Verification items for this drawing (mm, ordinates from the low corner). A direction names the side the tool comes from. Coordinates: 2 decimals unless noted, no trailing zeros. Order: outer loops, then holes, each group sorted by start corner. A loop starts at its lowest first (then second) coordinate and runs counter-clockwise, first axis right, second up. Notation, with made-up numbers: M 6,-8 L 48,-8 A14 ccw 48,16 Z; hole C 26,1.25 d7. An arc over 180 degrees is marked long. One line per item, written item: value. Start each with the question number.
1) Go/stop test with flat-tipped pins: P1, Ø6, axis at y = 17.5, z = 12.5, coming from the +X side; P2, Ø5, axis at x = 3, y = 5, coming from the +Z side; P3, Ø3, axis at y = 18.5, z = 7, coming from the -X side. Record where each tip stops, or that it passes through.
2) Sectioned sample at C-C, the plane y = 15. Enter the section's corners in (x, z).
3) Access from +Z, -Z, +X, -X, +Y, -Y to the whole of each face (thin tool, end or side, straight path). Record for the marked faces 1, 2, 3, 4 and 5.
4) Sectioned sample at A-A, the plane y = 31. Enter the section's corners in (x, z), then the cut area to 3 significant figures.
5) Draft check along X on the marked faces 6, 7 and 8. Enter one of: pulls with the +X half, pulls with the -X half, needs draft (parallel to the pull), parting line crosses it, or undercut.
6) Sectioned sample at B-B, the plane x = 3. Enter the section's corners in (y, z), then the cut area to 3 significant figures.
7) Thickness scan on L1, parallel to Y at x = 34, z = 0.8; L2, parallel to X at y = 2, z = 19; L3, parallel to X at y = 2, z = 2. Record the ranges inside material, lowest first. Write a range as from..to.
8) Sectioned sample at D-D, the plane z = 6.25. Enter the section's corners in (x, y), then the cut area to 3 significant figures.
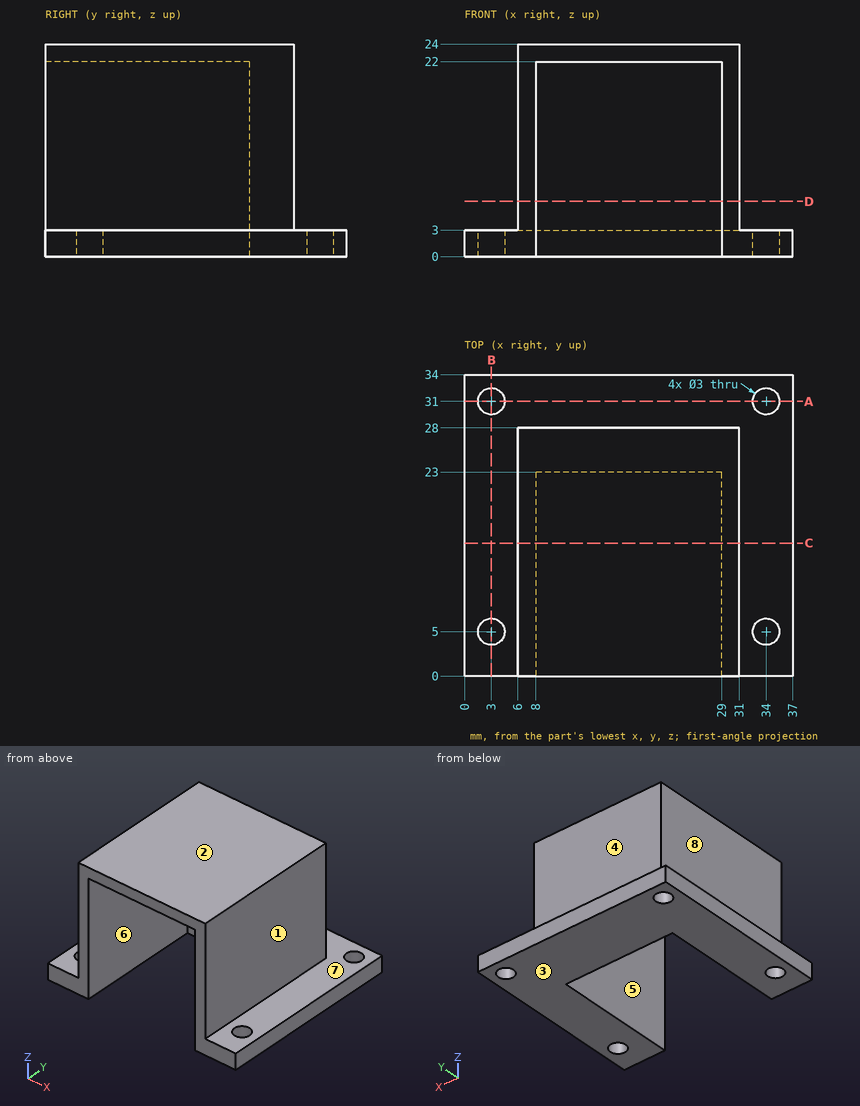
Final values:
1. P1: stops at x = 31
1. P2: stops at z = 3
1. P3: stops at x = 6
2. outline: M 0,0 L 8,0 L 8,22 L 29,22 L 29,0 L 37,0 L 37,3 L 31,3 L 31,24 L 6,24 L 6,3 L 0,3 Z
3. face 1: +Z, +X, +Y, -Y
3. face 2: +Z, +X, -X, +Y, -Y
3. face 3: -Z, +X, -X, +Y, -Y
3. face 4: +Z, +X, -X, +Y
3. face 5: -Z, -Y
4. outline: M 0,0 L 1.5,0 L 1.5,3 L 0,3 Z; M 4.5,0 L 32.5,0 L 32.5,3 L 4.5,3 Z; M 35.5,0 L 37,0 L 37,3 L 35.5,3 Z
4. area: 93.0 mm^2
5. face 6: undercut
5. face 7: needs draft
5. face 8: pulls with the -X half
6. outline: M 0,0 L 3.5,0 L 3.5,3 L 0,3 Z; M 6.5,0 L 29.5,0 L 29.5,3 L 6.5,3 Z; M 32.5,0 L 34,0 L 34,3 L 32.5,3 Z
6. area: 84.0 mm^2
7. L1: y = 0..3.5, 6.5..29.5, 32.5..34
7. L2: x = 6..8, 29..31
7. L3: x = 0..8, 29..37
8. outline: M 6,0 L 8,0 L 8,23 L 29,23 L 29,0 L 31,0 L 31,28 L 6,28 Z
8. area: 217 mm^2
